Check sheet for the modelled part. Datum: model origin and axes. Units: mm. Round coordinates to 2 decimals unless told otherwise and drop trailing zeros. Loops run counter-clockwise (first coordinate to the right, second up) from the corner with the lowest first, then second, coordinate; pieces in that order, holes last. Notation, with made-up numbers: (-1.5, 3.5) - (51.5, 3.5) arc R26 ccw to (51.5, 29.5) - close; hole circle Ø4 at (49, 46). An arc over 180 degrees is marked (long way). Put each result on its own line as item: value. Start each with the question number.
Item 1: Section check C-C, the plane y = 8.5. Record the cut outline in (x, z).
Item 2: Section check B-B, the plane z = 0. Record the cut outline in (x, y), and give its area (3 significant figures).
Item 3: Gauge pin test, flat ends, axial feed: pin 1 Ø3 at (y, z) = (20.5, 14) entering from -X; pin 2 Ø1 at (y, z) = (23, -10.5) entering from +X; pin 3 Ø8 at (x, y) = (15, 11.5) entering from +Z; pin 4 Ø8 at (x, z) = (-13.5, 9) entering from -Y. Record the tip position at first contact, or that the pin passes through.
Item 4: Section check A-A, the plane x = 0. Record the cut outline in (y, z), and give its area (3 significant figures).
Item 5: Material ranges on line 1 along X through (y, z) = (9, 0); line 2 along Z through (x, y) = (4.5, 28.75), recorded low to high.
Item 6: Draft check along Z on faces 1 (the flat face through (8, 0, -9)), 2 (the cylindrical face through (-5.78, 15.2, -7.54)), 3 (the flat face through (0, 15, 19.401)), 4 (the flat face through (-13.643, 14.79, -13.794)). Enter one of: pulls with the +Z half, pulls with the -Z half, needs draft (parallel to the pull), parting line crosses it, or undercut.
Item 7: Section check D-D, the plane x = 15. Record the cut outline in (y, z), and give its area (3 significant figures).
from build123d import *

# Parameters (mm, degrees)
BOSS_EXTRUDE1_DEPTH = 30
SKETCH3_R           = 9.5
CUT_EXTRUDE1_DEPTH  = 41.655062299
CHAMFER1_SIZE       = 1
FILLET1_R           = 1


with BuildPart() as part:
    # Sketch2 → Boss-Extrude1 (new body)
    with BuildSketch(Plane(origin=(0, 0, 0), x_dir=(1, 0, 0), z_dir=(0, 1, 0))):
        Polygon((19.401470183, -8.03635208), (19.401470183, 8.03635208), (8.03635208, 19.401470183), (-8.03635208, 19.401470183), (-19.401470183, 8.03635208), (-19.401470183, -8.03635208), (-8.03635208, -19.401470183), (8.03635208, -19.401470183), align=None)
    extrude(amount=BOSS_EXTRUDE1_DEPTH)

    # Sketch3 → Cut-Extrude1 (cut, through all)
    with BuildSketch(Plane(origin=(0, 30, 0), x_dir=(1, 0, 0), z_dir=(0, 1, 0))):
        with Locations(Location((0, 0, 0), (0, 0, 270))):
            Circle(SKETCH3_R)
    extrude(amount=-CUT_EXTRUDE1_DEPTH, mode=Mode.SUBTRACT)

    # Chamfer1
    chamfer1_edges = [part.edges().sort_by_distance(p)[0] for p in [
        (0, 0, -9.5),
        (0, 30, -9.5),
    ]]
    chamfer(chamfer1_edges, length=CHAMFER1_SIZE)

    # Fillet1
    fillet1_edges = [part.edges().sort_by_distance(p)[0] for p in [
        (19.401470183, 15, -8.03635208),
        (19.401470183, 15, 8.03635208),
        (8.03635208, 15, 19.401470183),
        (-8.03635208, 15, 19.401470183),
        (-19.401470183, 15, 8.03635208),
        (-19.401470183, 15, -8.03635208),
        (-8.03635208, 15, -19.401470183),
        (8.03635208, 15, -19.401470183),
    ]]
    fillet(fillet1_edges, radius=FILLET1_R)


solid = part.part
Check result:
1. outline: (-19.4, -7.62) arc R1 ccw to (-19.11, -8.33) - (-8.33, -19.11) arc R1 ccw to (-7.62, -19.4) - (7.62, -19.4) arc R1 ccw to (8.33, -19.11) - (19.11, -8.33) arc R1 ccw to (19.4, -7.62) - (19.4, 7.62) arc R1 ccw to (19.11, 8.33) - (8.33, 19.11) arc R1 ccw to (7.62, 19.4) - (-7.62, 19.4) arc R1 ccw to (-8.33, 19.11) - (-19.11, 8.33) arc R1 ccw to (-19.4, 7.62) - close; hole circle Ø19 at (0, 0)
2. outline: (-19.4, 0) - (-10.5, 0) - (-9.5, 1) - (-9.5, 29) - (-10.5, 30) - (-19.4, 30) - close; (9.5, 1) - (10.5, 0) - (19.4, 0) - (19.4, 30) - (10.5, 30) - (9.5, 29) - close
2. area: 592 mm²
3. pin 1: x = -14.94
3. pin 2: x = 17.44
3. pin 3: z = 16.44
3. pin 4: y = 0
4. outline: (0, -19.4) - (30, -19.4) - (30, -10.5) - (29, -9.5) - (1, -9.5) - (0, -10.5) - close; (0, 10.5) - (1, 9.5) - (29, 9.5) - (30, 10.5) - (30, 19.4) - (0, 19.4) - close
4. area: 592 mm²
5. line 1: -19.4 to -9.5, 9.5 to 19.4
5. line 2: -19.4 to -8.37, 8.37 to 19.4
6. face 1: needs draft
6. face 2: undercut
6. face 3: pulls with the +Z half
6. face 4: pulls with the -Z half
7. outline: (0, -12.44) - (30, -12.44) - (30, 12.44) - (0, 12.44) - close
7. area: 746 mm²
